Answer from the drawing. Dimensions are ordinates in mm from the lowest x, y and z of the part. A direction names the side the tool comes from. Give positions to 0.01 mm unless a question says otherwise; leave off trailing zeros. Loops run counter-clockwise (first coordinate to the right, second up) from the corner with the lowest first, then second, coordinate; pieces in that order, holes last. Notation, with made-up numbers: (18, 53) - (42, 53) arc R12 ccw to (42, 70) - close; hole circle Ø11 at (10, 29). An arc over 180 degrees is marked (long way). Answer as CSV lines item,"result". Start each with the question number.
1) A cutting plane is placed at D-D (y = 10.75). Determine the outline of the cut face in (x, z), and give its area (3 significant figures).
2) For the marked faces 1, 2, 3 and 4, determine the directions among +Z, -Z, +X, -X, +Y, -Y from which every point of the face is accessible in a straight line to the end or side of a thin tool.
3) Flat-ended cylindrical pins translate along their axes: pin 1 (3 mm diameter, centred on y = 14, z = 35.5, fed in from -X); pin 2 (1.5 mm diameter, centred on x = 13.5, y = 6, fed in from +Z); pin 3 (2.5 mm diameter, centred on x = 18.5, z = 41, fed in from -Y). Find the tip coordinate at first contact, or state that the pin passes through.
4) Find the intervals of material crossed by line 1 along Z through (x, y) = (18.1, 15); line 2 along Z through (x, y) = (19, 20.75); line 3 along X through (y, z) = (10.25, 44), in increasing order.
5) A cutting plane is placed at A-A (y = 15). Determine the outline of the cut face in (x, z).
6) A cutting plane is placed at C-C (x = 19). Determine the outline of the cut face in (y, z).
7) A cutting plane is placed at B-B (z = 45). Determine the outline of the cut face in (x, y), and give its area (3 significant figures).
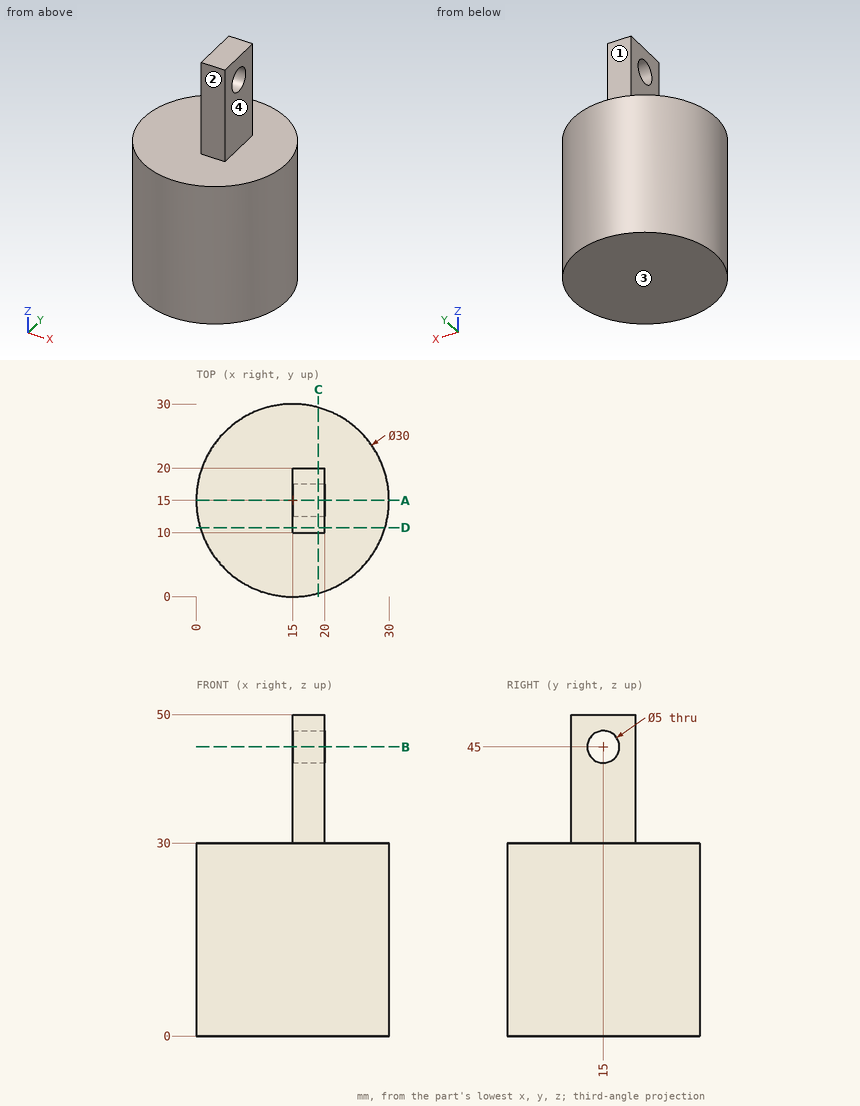
Ans:
1,outline,"(0.61, 0) - (29.39, 0) - (29.39, 30) - (20, 30) - (20, 50) - (15, 50) - (15, 30) - (0.61, 30) - close"
1,area,"963 mm2"
2,face 1,"+Z, +X, -X, +Y"
2,face 2,"+Z, +X, -X, -Y"
2,face 3,"-Z, +X, -X, +Y, -Y"
2,face 4,"+Z, +X, +Y, -Y"
3,pin 1,"x = 15"
3,pin 2,"z = 30"
3,pin 3,"y = 10"
4,line 1,"0 to 42.5, 47.5 to 50"
4,line 2,"0 to 30"
4,line 3,"15 to 20"
5,outline,"(0, 0) - (30, 0) - (30, 30) - (20, 30) - (20, 42.5) - (15, 42.5) - (15, 30) - (0, 30) - close; (15, 47.5) - (20, 47.5) - (20, 50) - (15, 50) - close"
6,outline,"(0.54, 0) - (29.46, 0) - (29.46, 30) - (20, 30) - (20, 50) - (10, 50) - (10, 30) - (0.54, 30) - close; hole circle Ø5 at (15, 45)"
7,outline,"(15, 10) - (20, 10) - (20, 12.5) - (15, 12.5) - close; (15, 17.5) - (20, 17.5) - (20, 20) - (15, 20) - close"
7,area,"25.0 mm2"
